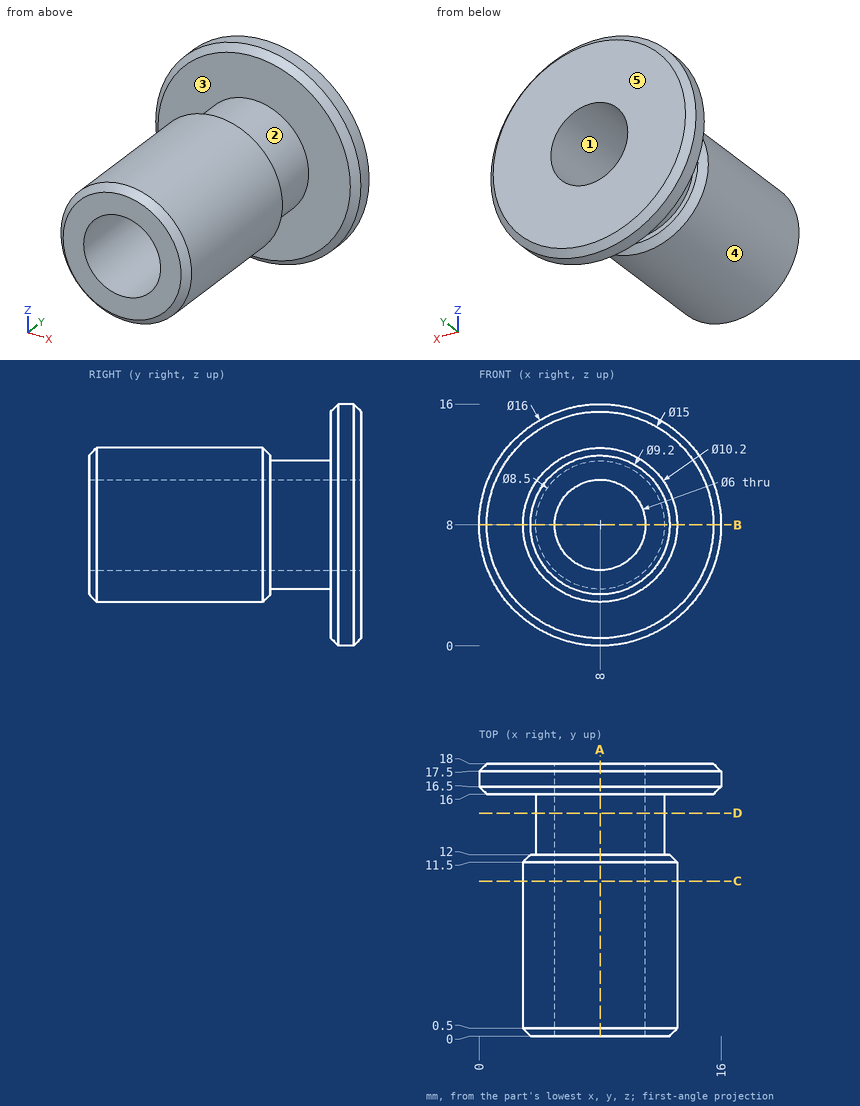
Check sheet for the drawn part. Datum: minimum x, y, z corner. Units: mm. A direction names the side the tool comes from. Give positions to 0.01 mm unless a question says otherwise; leave off trailing zeros. Order: outer loops, then holes, each group sorted by start corner. A loop starts at its lowest first (then second) coordinate and runs counter-clockwise, first axis right, second up. Notation, with made-up numbers: (71.5, 79) -> (99.5, 79) arc R18 cw to (99.5, 112) -> close; hole circle Ø6 at (19, -27.75). An arc over 180 degrees is marked (long way). Answer as CSV lines item,"result".
Q1. Sectioned sample at B-B on z = 8. Record the cut outline in (x, y).
Solutions:
outline,"(0, 16.5) -> (0.5, 16) -> (3.75, 16) -> (3.75, 12) -> (3.4, 12) -> (2.9, 11.5) -> (2.9, 0.5) -> (3.4, 0) -> (5, 0) -> (5, 18) -> (0.5, 18) -> (0, 17.5) -> close; (11, 0) -> (12.6, 0) -> (13.1, 0.5) -> (13.1, 11.5) -> (12.6, 12) -> (12.25, 12) -> (12.25, 16) -> (15.5, 16) -> (16, 16.5) -> (16, 17.5) -> (15.5, 18) -> (11, 18) -> close"
Q2. Sectioned sample at C-C on y = 10.25. Record the cut outline in (x, z).
Solutions:
outline,"circle Ø10.2 at (8, 8); hole circle Ø6 at (8, 8)"
Q3. Depth check by flat-ended pin: pin 1 (8 mm diameter, centred on y = 6.5, z = 7, fed in from +X); pin 2 (8 mm diameter, centred on y = 6.5, z = 9, fed in from -X); pin 3 (3 mm diameter, centred on y = 15, z = 6.5, fed in from -X). Enter the tip coordinate at first touch or a pass-through.
Solutions:
pin 1,"stops at x = 13.1"
pin 2,"stops at x = 2.9"
pin 3,"stops at x = 0.12"
Q4. Sectioned sample at D-D on y = 14.75. Record the cut outline in (x, z), plus the area to 3 significant figures.
Solutions:
outline,"circle Ø8.5 at (8, 8); hole circle Ø6 at (8, 8)"
area,"28.5 mm²"
Q5. Access from +Z, -Z, +X, -X, +Y, -Y to the whole of each face (thin tool, end or side, straight path). Record for the marked faces 4 and 5.
Solutions:
face 4,"-Y"
face 5,"+Z, -Z, +X, -X, +Y"
Q6. Sectioned sample at A-A on x = 8. Record the cut outline in (y, z), plus the area to 3 significant figures.
Solutions:
outline,"(0, 3.4) -> (0.5, 2.9) -> (11.5, 2.9) -> (12, 3.4) -> (12, 3.75) -> (16, 3.75) -> (16, 0.5) -> (16.5, 0) -> (17.5, 0) -> (18, 0.5) -> (18, 5) -> (0, 5) -> close; (0, 11) -> (18, 11) -> (18, 15.5) -> (17.5, 16) -> (16.5, 16) -> (16, 15.5) -> (16, 12.25) -> (12, 12.25) -> (12, 12.6) -> (11.5, 13.1) -> (0.5, 13.1) -> (0, 12.6) -> close"
area,"79.4 mm²"
Q7. Scan lines: probe 1 along Z at (x, y) = (8, 9.5); probe 2 along Z at (x, y) = (8, 13.5); probe 3 along Y at (x, z) = (2, 4). Record each from-to range of solid material in increasing order.
Solutions:
probe 1,"z = 2.9 to 5, 11 to 13.1"
probe 2,"z = 3.75 to 5, 11 to 12.25"
probe 3,"y = 16 to 18"
Q8. Release check for a two-part mould opening along Z. For the marked faces 1, 2 and 3 record: +Z half, -Z half, draft (parallel to the pull), parting line (faces both ways), or undercut.
Solutions:
face 1,"undercut"
face 2,"parting line"
face 3,"draft"
